Job drawing, mm, ordinate dimensions from the low corner. One solid piece. A direction names the side the tool comes from. Give positions to 0.01 mm unless a question says otherwise; leave off trailing zeros. Write each loop counter-clockwise with the first axis right and the second up, starting at its lowest first coordinate (ties: lowest second). Pieces come first, ordered by that corner, then holes. Notation, with made-up numbers: M 41.5,18.5 L 60.5,18.5 A31 cw 60.5,49.5 Z; hole C 5.25,-26 d9. An arc over 180 degrees is marked long. Answer as CSV lines item,"result". Start each with the question number.
1) Mould opens along Y. For the marked faces 3, 4 and 5 say: pulls with the +Y half, pulls with the -Y half, needs draft (parallel to the pull), parting line crosses it, or undercut.
2) Slice it at B-B, the plane x = 196.5. Give the cut face in (y, z).
3) Slice it at A-A, the plane z = 196.5. Give the cut face in (x, y), plus the area to 3 significant figures.
4) Slice it at C-C, the plane z = 70.5. Give the cut face in (x, y), plus the area to 3 significant figures.
5) Slice it at D-D, the plane y = 182.5. Give the cut face in (x, z), plus the area to 3 significant figures.
6) Tool access for the marked faces 1 and 2: list every direction of +Z, -Z, +X, -X, +Y, -Y with a clear straight run to the whole face (end or side of a thin tool).
7) Wall check: line 1 along X through (y, z) = (252, 190); line 2 along Z through (x, y) = (194.5, 306). Give the ranges that are in metal, low to high. Write a range as from..to.
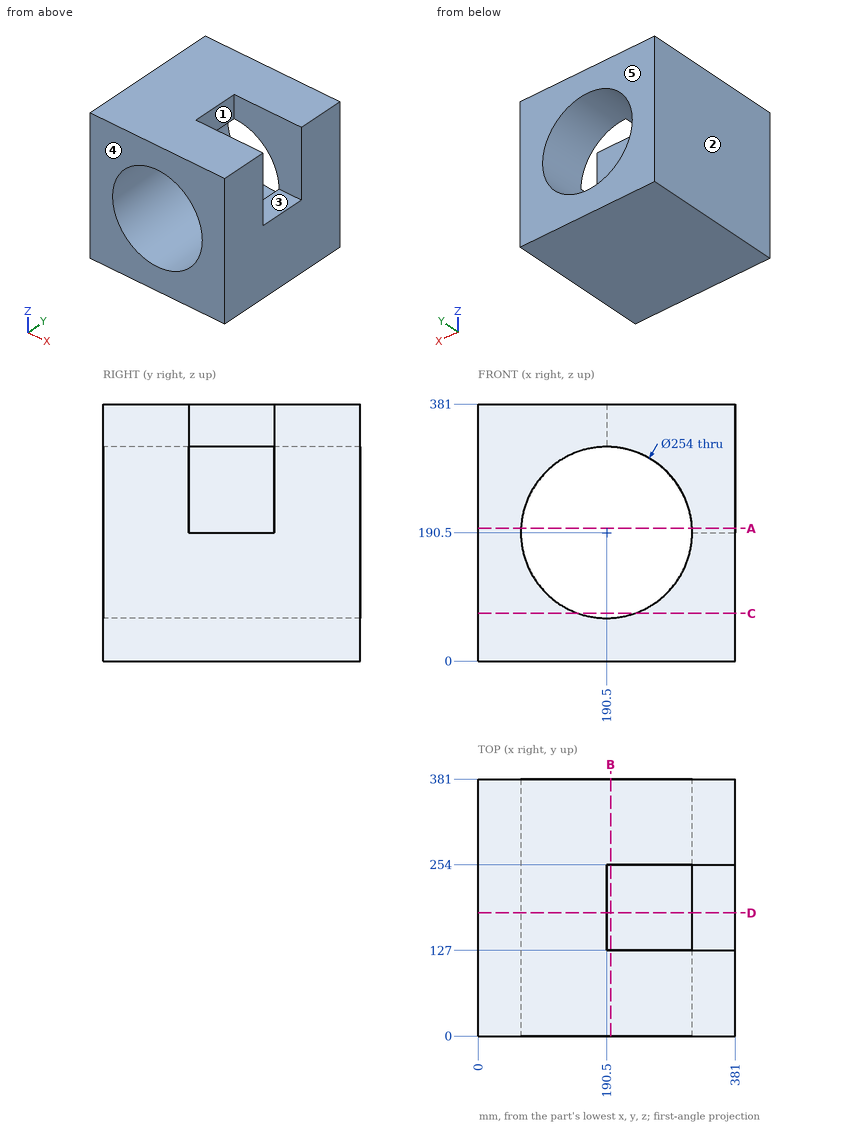
Found:
1,face 3,"undercut"
1,face 4,"pulls with the -Y half"
1,face 5,"pulls with the +Y half"
2,outline,"M 0,0 L 381,0 L 381,63.64 L 0,63.64 Z; M 0,317.36 L 127,317.36 L 127,381 L 0,381 Z; M 254,317.36 L 381,317.36 L 381,381 L 254,381 Z"
3,outline,"M 0,0 L 63.64,0 L 63.64,381 L 0,381 Z; M 317.36,0 L 381,0 L 381,127 L 317.36,127 Z; M 317.36,254 L 381,254 L 381,381 L 317.36,381 Z"
3,area,"40,400 mm²"
4,outline,"M 0,0 L 148.92,0 L 148.92,381 L 0,381 Z; M 232.08,0 L 381,0 L 381,381 L 232.08,381 Z"
4,area,"113,000 mm²"
5,outline,"M 0,0 L 381,0 L 381,190.5 L 317.5,190.5 A127 cw long 190.5,317.5 L 190.5,381 L 0,381 Z"
5,area,"70,900 mm²"
6,face 1,"+Z, +X"
6,face 2,"+Z, -Z, -X, +Y, -Y"
7,line 1,"0..63.5, 317.5..381"
7,line 2,"0..63.56, 317.44..381"
